Job drawing, mm, ordinate dimensions from the low corner. One solid piece. A direction names the side the tool comes from. Give positions to 0.01 mm unless a question says otherwise; leave off trailing zeros. Order: outer loops, then holes, each group sorted by start corner. A loop starts at its lowest first (then second) coordinate and runs counter-clockwise, first axis right, second up. Notation, with made-up numbers: (86, 1.25) - (131, 1.25) arc R18 ccw to (131, 20.25) - close; hole circle Ø9 at (28, 20.5). An arc over 180 degrees is marked (long way). Use one line per item in the form item = value. Start each with the question number.
1. Band-saw the part on A-A, the plane z = 12.7. List the corners of the cut face in (x, y) (3 decimals), plus the area to 3 significant figures.
2. Pin check, flat tips, straight feed: P1, Ø1, axis at x = 11.5, z = 19.5, coming from the +Y side (3 decimals); P2, Ø11, axis at x = 17.5, y = 17, coming from the +Z side (3 decimals); P3, Ø4, axis at y = 13.5, z = 6, coming from the +X side. Stop position of each tip, or through.
3. Tool access for the marked faces 1 and 2: list every direction of +Z, -Z, +X, -X, +Y, -Y with a clear straight run to the whole face (end or side of a thin tool).
4. Band-saw the part on D-D, the plane y = 2.5. List the corners of the cut face in (x, z).
5. Drill centre lines: line 1 (Y direction, x = 12.7, z = 2.5); line 2 (Z direction, x = 12.7, y = 1.6); line 3 (X direction, y = 19.05, z = 1.15). Where is each one in solid material? Low to high.
6. Band-saw the part on C-C, the plane x = 12.7. State how many separate pieces and enclosed holes the cut face has, plus the area to 3 significant figures.
7. Band-saw the part on B-B, the plane y = 19.05. List the corners of the cut face in (x, z) (1 decimal).
8. Pull direction X, two halves, no side cores. Call the marked faces 3, 4 and 5: +X half, -X half, draft (parallel to the pull), parting line (faces both ways), or undercut.
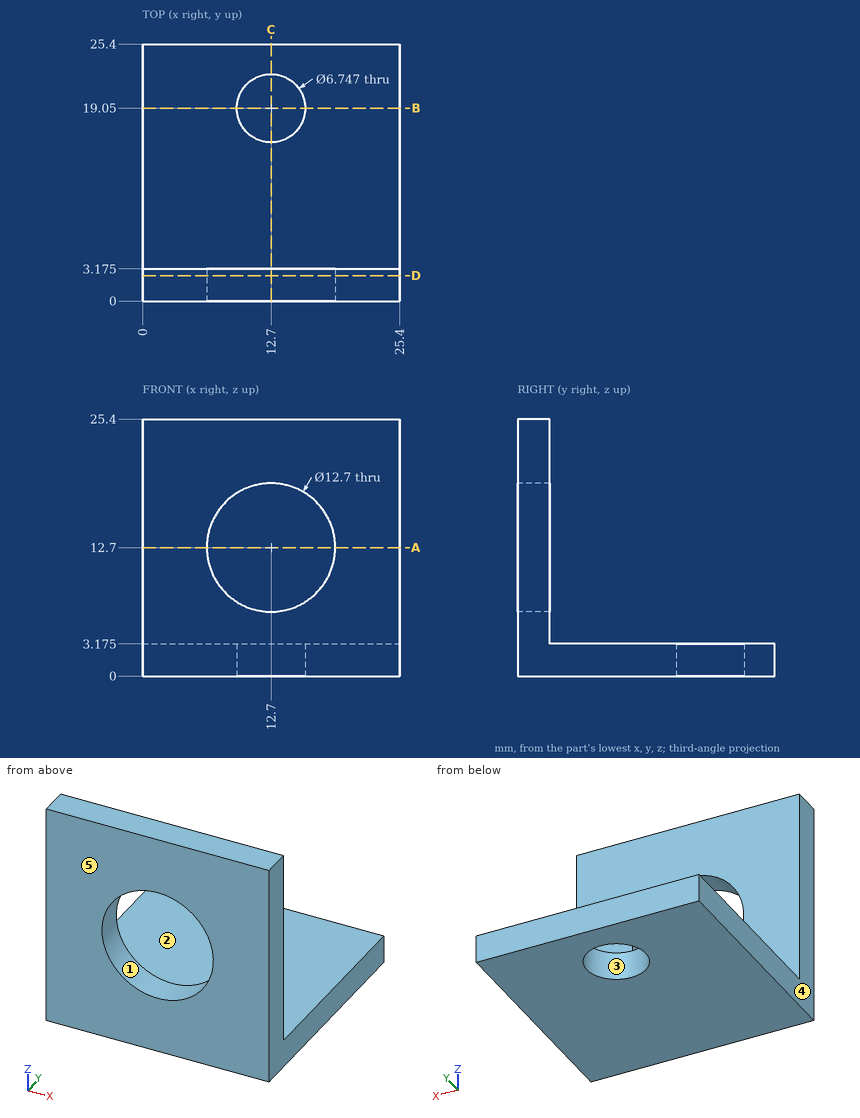
From the geometry:
q1.outline = (0, 0) - (6.35, 0) - (6.35, 3.175) - (0, 3.175) - close; (19.05, 0) - (25.4, 0) - (25.4, 3.175) - (19.05, 3.175) - close
q1.area = 40.3 mm²
q2.P1 = 3.175
q2.P2 = 3.175
q2.P3 = through
q3.face_1 = +Y, -Y
q3.face_2 = +Z, +X, -X, +Y
q4.outline = (0, 0) - (25.4, 0) - (25.4, 25.4) - (0, 25.4) - close; hole circle Ø12.7 at (12.7, 12.7)
q5.line_1 = 0 to 15.68, 22.42 to 25.4
q5.line_2 = 0 to 6.35, 19.05 to 25.4
q5.line_3 = 0 to 9.33, 16.07 to 25.4
q6.separate_pieces = 3
q6.enclosed_holes = 0
q6.area = 89.5 mm²
q7.outline = (0, 0) - (9.3, 0) - (9.3, 3.2) - (0, 3.2) - close; (16.1, 0) - (25.4, 0) - (25.4, 3.2) - (16.1, 3.2) - close
q8.face_3 = undercut
q8.face_4 = -X half
q8.face_5 = draft
